The model under review builds one solid part; all positions refer to its coordinate system, in mm. Give positions to 0.01 mm unless a question says otherwise; leave off trailing zeros. Loops run counter-clockwise (first coordinate to the right, second up) from the corner with the lowest first, then second, coordinate; pieces in that order, holes last. Notation, with made-up numbers: M 38.25,83 L 49.25,83 A24 ccw 49.25,118 Z; hole C -17,-16 d7. An arc over 180 degrees is marked long. One line per item, written item: value. Start each with the question number.
Q1. For pin 1 (2.5 mm diameter, centred on y = 40, z = 3, fed in from -X); pin 2 (18 mm diameter, centred on x = 0, y = 0, fed in from -Z); pin 3 (16 mm diameter, centred on x = 58.16, y = 0, fed in from -Z); pin 4 (1.5 mm diameter, centred on x = 32.5, z = 1.5, fed in from -Y), all flat-tipped, find the tip position at first contact; note any pin that passes through.
Q2. To check wall thickness, follow line 1 along Y through (x, z) = (0, 3.5); line 2 along Y through (x, z) = (-53, 3.2); line 3 along Y through (x, z) = (-19, 0.4). State the ranges of each line that lie inside material, in increasing order. Write a range as from..to.
Q3. We need section C-C on x = 18. Write out the cut boundary in (y, z).
Q4. We need section D-D on y = -39. Write out the cut boundary in (x, z).
Q5. We need section A-A on x = 0. Write out the cut boundary in (y, z), plus the area to 3 significant figures.
```python
from build123d import *

# Parameters (mm, degrees)
SKETCH1_R           = 75
SKETCH1_R_2         = 15
BOSS_EXTRUDE1_DEPTH = 5
SKETCH2_R           = 5
CUT_EXTRUDE1_DEPTH  = 5
CUT_EXTRUDE2_DEPTH  = 5
FILLET1_R           = 13
FILLET2_R           = 8


with BuildPart() as part:
    # Sketch1 → Boss-Extrude1 (new body)
    with BuildSketch(Plane.XY):
        Circle(SKETCH1_R)
        Circle(SKETCH1_R_2, mode=Mode.SUBTRACT)
    extrude(amount=BOSS_EXTRUDE1_DEPTH)

    # Sketch2 → Cut-Extrude1 (cut)
    with BuildSketch(Plane.XY.offset(5)):
        with BuildLine():
            Line((-10, -64.226162893), (-10, -17.320508076))
            ThreePointArc((-10, -17.320508076), (-14.142135624, -14.142135624), (-17.320508076, -10))
            Line((-17.320508076, -10), (-64.226162893, -10))
            ThreePointArc((-64.226162893, -10), (-45.961940777, -45.961940777), (-10, -64.226162893))
        make_face()
        with BuildLine():
            Line((-64.226162893, 10), (-17.320508076, 10))
            ThreePointArc((-17.320508076, 10), (-14.142135624, 14.142135624), (-10, 17.320508076))
            Line((-10, 17.320508076), (-10, 64.226162893))
            ThreePointArc((-10, 64.226162893), (-45.961940777, 45.961940777), (-64.226162893, 10))
        make_face()
        with BuildLine():
            Line((10, 64.226162893), (10, 17.320508076))
            ThreePointArc((10, 17.320508076), (14.142135624, 14.142135624), (17.320508076, 10))
            Line((17.320508076, 10), (64.226162893, 10))
            ThreePointArc((64.226162893, 10), (45.961940777, 45.961940777), (10, 64.226162893))
        make_face()
        with Locations((58.156758338, 0)):
            Circle(SKETCH2_R)
        with Locations((0, -58.156758338)):
            Circle(SKETCH2_R)
        with Locations((-58.156758338, 0)):
            Circle(SKETCH2_R)
        with Locations((0, 58.156758338)):
            Circle(SKETCH2_R)
    extrude(amount=-CUT_EXTRUDE1_DEPTH, mode=Mode.SUBTRACT)

    # Sketch2_3 → Cut-Extrude2 (cut)
    with BuildSketch(Plane.XY.offset(5)):
        with BuildLine():
            Line((17.320508076, -10), (64.226162893, -10))
            ThreePointArc((64.226162893, -10), (45.961940777, -45.961940777), (10, -64.226162893))
            Line((10, -64.226162893), (10, -17.320508076))
            ThreePointArc((10, -17.320508076), (14.142135624, -14.142135624), (17.320508076, -10))
        make_face()
    extrude(amount=-CUT_EXTRUDE2_DEPTH, mode=Mode.SUBTRACT)

    # Fillet1
    fillet1_edges = [part.edges().sort_by_distance(p)[0] for p in [
        (10, 17.320508076, 2.5),
        (17.320508076, 10, 2.5),
        (-10, -17.320508076, 2.5),
        (-17.320508076, -10, 2.5),
        (-17.320508076, 10, 2.5),
        (-10, 17.320508076, 2.5),
        (17.320508076, -10, 2.5),
        (10, -17.320508076, 2.5),
    ]]
    fillet(fillet1_edges, radius=FILLET1_R)

    # Fillet2
    fillet2_edges = [part.edges().sort_by_distance(p)[0] for p in [
        (10, 64.226162893, 2.5),
        (64.226162893, 10, 2.5),
        (-10, -64.226162893, 2.5),
        (-64.226162893, -10, 2.5),
        (-64.226162893, 10, 2.5),
        (-10, 64.226162893, 2.5),
        (64.226162893, -10, 2.5),
        (10, -64.226162893, 2.5),
    ]]
    fillet(fillet2_edges, radius=FILLET2_R)


solid = part.part
```
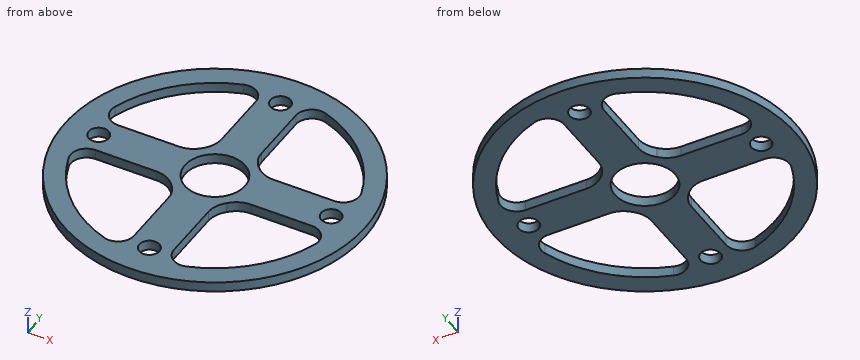
Solved:
1. pin 1: x = -64.21
1. pin 2: through
1. pin 3: z = 0
1. pin 4: y = -67.95
2. line 1: -75..-63.16, -53.16..-15, 15..53.16, 63.16..75
2. line 2: -53.07..-37.63, -10..10, 37.63..53.07
2. line 3: -72.55..-62.02, -10.87..10.87, 62.02..72.55
3. outline: M -72.81,0 L -62.08,0 L -62.08,5 L -72.81,5 Z; M -11.3,0 L 11.3,0 L 11.3,5 L -11.3,5 Z; M 62.08,0 L 72.81,0 L 72.81,5 L 62.08,5 Z
4. outline: M -64.06,0 L -52,0 L -52,5 L -64.06,5 Z; M -10,0 L 10,0 L 10,5 L -10,5 Z; M 52,0 L 64.06,0 L 64.06,5 L 52,5 Z
5. outline: M -75,0 L -63.16,0 L -63.16,5 L -75,5 Z; M -53.16,0 L -15,0 L -15,5 L -53.16,5 Z; M 15,0 L 53.16,0 L 53.16,5 L 15,5 Z; M 63.16,0 L 75,0 L 75,5 L 63.16,5 Z
5. area: 500 mm2
